Autodesk Inventor part; units mm, degrees
ref_plane "YZ Plane" through (0, 0, 0) normal (1, 0, 0) x (0, 1, 0)
ref_plane "XZ Plane" through (0, 0, 0) normal (0, 1, 0) x (-1, 0, 0)
ref_plane "XY Plane" through (0, 0, 0) normal (0, 0, 1) x (1, 0, 0)
sketch "Sketch1" plane through (0, 0, 0) normal (0, 0, 1) x (1, 0, 0)
  line L0 (0, 7.3323) -> (6.35, 3.6662)
  line L1 (6.35, 3.6662) -> (6.35, -3.6662)
  line L2 (6.35, -3.6662) -> (0, -7.3323)
  line L3 (0, -7.3323) -> (-6.35, -3.6662)
  line L4 (-6.35, -3.6662) -> (-6.35, 3.6662)
  line L5 (-6.35, 3.6662) -> (0, 7.3323)
  point P0 (0, 0)
  point P1 (0, 0)
  dimension "d0" = 12.7
extrude "Extrusion1" add sketch "Sketch1" along normal mid plane 63.5
sketch "Sketch4" plane through (0, 0, 31.75) normal (0, 0, 1) x (1, 0, 0)
  circle A0 centre (0, 0) radius 4.7625
  line L0 (-6.35, 3.6662) -> (-6.35, -3.6662)
  line L1 (-6.35, -3.6662) -> (0, -7.3323)
  line L2 (0, -7.3323) -> (6.35, -3.6662)
  line L3 (6.35, -3.6662) -> (6.35, 3.6662)
  line L4 (6.35, 3.6662) -> (0, 7.3323)
  line L5 (0, 7.3323) -> (-6.35, 3.6662)
  dimension "d7" = 9.525
extrude "Extrusion2" cut sketch "Sketch4" against normal blind 7.1374
mirror "Mirror1" about plane through (0, 0, 0) normal (0, 0, 1) of "Extrusion2"
properties part number "GearShaft" material "Steel, Alloy"
Verification items for the finished model (mm, model axes). A direction names the side the tool comes from. Coordinates: 2 decimals unless noted, no trailing zeros. Order: outer loops, then holes, each group sorted by start corner. A loop starts at its lowest first (then second) coordinate and runs counter-clockwise, first axis right, second up. Notation, with made-up numbers: (-35, -22) -> (0, -22) arc R16 ccw to (0, -5) -> close; hole circle Ø3 at (-9, 76.5). An arc over 180 degrees is marked (long way). Answer as CSV lines item,"result". Start each with the question number.
1) Cross-section at D-D, the plane y = 6.25. Record the boundary of the cut face in (x, z).
2) Cross-section at B-B, the plane z = 3.5. Record the boundary of the cut face in (x, y), then the cut area to 3 significant figures.
3) Set-up check for faces 1 (the face through (0, -5, -24.613)), 2 (the face through (-3.219, 5.474, -0.345)), 3 (the face through (0, -5, 24.613)): record each of +Z, -Z, +X, -X, +Y, -Y from which the full face is reachable in a straight line by a thin tool's end or side.
4) Gauge pin test, flat ends, axial feed: pin 1 Ø4 at (x, z) = (-3.5, 1) entering from +Y; pin 2 Ø4 at (x, z) = (2.5, 12) entering from +Y; pin 3 Ø1.5 at (x, z) = (-2, -5.5) entering from -Y. Record the tip position at first contact, or that the pin passes through.
5) Material ranges on L1, parallel to Z at x = 5, y = 1; L2, parallel to Y at x = 3.75, z = 3; L3, parallel to Y at x = 1, z = 25, recorded low to high. Write a range as [from, to].
6) Cross-section at A-A, the plane y = 0. Record the boundary of the cut face in (x, z), then the cut area to 3 significant figures.
7) Cross-section at C-C, the plane x = -3.5. Record the boundary of the cut face in (y, z).
Conclusion:
1,outline,"(-1.87, -24.61) -> (1.87, -24.61) -> (1.87, 24.61) -> (-1.87, 24.61) -> close"
2,outline,"(-6.35, -3.67) -> (0, -7.33) -> (6.35, -3.67) -> (6.35, 3.67) -> (0, 7.33) -> (-6.35, 3.67) -> close"
2,area,"140 mm²"
3,face 1,"-Z"
3,face 2,"+Z, -Z, -X, +Y"
3,face 3,"+Z"
4,pin 1,"stops at y = 6.47"
4,pin 2,"stops at y = 7.04"
4,pin 3,"stops at y = -6.61"
5,L1,"z = [-24.61, 24.61]"
5,L2,"y = [-5.17, 5.17]"
5,L3,"y = [-4.66, 4.66]"
6,outline,"(-6.35, -24.61) -> (-4.76, -24.61) -> (-4.76, -31.75) -> (4.76, -31.75) -> (4.76, -24.61) -> (6.35, -24.61) -> (6.35, 24.61) -> (4.76, 24.61) -> (4.76, 31.75) -> (-4.76, 31.75) -> (-4.76, 24.61) -> (-6.35, 24.61) -> close"
6,area,"761 mm²"
7,outline,"(-5.31, -24.61) -> (-3.23, -24.61) -> (-3.23, -31.75) -> (3.23, -31.75) -> (3.23, -24.61) -> (5.31, -24.61) -> (5.31, 24.61) -> (3.23, 24.61) -> (3.23, 31.75) -> (-3.23, 31.75) -> (-3.23, 24.61) -> (-5.31, 24.61) -> close"
